from build123d import *

# Parameters (mm, degrees)
PROTO_PENTAGRAM_R   = 7.5
PROTO_PENTAGRAM_R_2 = 2.5
BOSS_EXTRUDE1_DEPTH = 15
PICK_1_R            = 1.85
CUT_EXTRUDE1_DEPTH  = 15
PICK_2_R            = 1.85
CUT_EXTRUDE2_DEPTH  = 15
PICK_3_R            = 1.85
CUT_EXTRUDE3_DEPTH  = 15
PICK_4_R            = 1.85
CUT_EXTRUDE4_DEPTH  = 15
PICK_5_R            = 1.85
CUT_EXTRUDE5_DEPTH  = 15
FILLET1_R           = 5


with BuildPart() as part:
    # proto-pentagram → Boss-Extrude1 (new body)
    # profile 1 of 2: a face of its own
    with BuildSketch(Plane(origin=(0, 0, 0), x_dir=(1, 0, 0), z_dir=(0, 1, 0))):
        Polygon((47.921856642, -22.405259561), (6.5, -8.946482483), (6.5, -52.5), (-6.5, -52.5), (-6.5, -8.946482483), (-47.921856642, -22.405259561), (-51.939077569, -10.041524849), (-10.517220927, 3.417252229), (-36.117336209, 38.652788065), (-25.600115282, 46.293996345), (0, 11.058460509), (25.600115282, 46.293996345), (36.117336209, 38.652788065), (10.517220927, 3.417252229), (51.939077569, -10.041524849), align=None)
        Circle(PROTO_PENTAGRAM_R, mode=Mode.SUBTRACT)
    # profile 2 of 2: a face of its own
    with BuildSketch(Plane(origin=(0, 0, 0), x_dir=(1, 0, 0), z_dir=(0, 1, 0))):
        Circle(PROTO_PENTAGRAM_R)
        with Locations(Location((0, 0, 0), (0, 0, 270))):
            Circle(PROTO_PENTAGRAM_R_2, mode=Mode.SUBTRACT)
    extrude(amount=BOSS_EXTRUDE1_DEPTH)

    # pick-1 → Cut-Extrude1 (cut)
    with BuildSketch(Plane(origin=(6.5, 0, 0), x_dir=(0, 0, -1), z_dir=(1, 0, 0))):
        with Locations((-46.5, 7.5)):
            Circle(PICK_1_R)
        with Locations((-32.5, 7.5)):
            Circle(PICK_1_R)
    extrude(amount=-CUT_EXTRUDE1_DEPTH, mode=Mode.SUBTRACT)

    # pick-2 → Cut-Extrude2 (cut)
    with BuildSketch(Plane(origin=(2.008610463, 0, -6.181867356), x_dir=(-0.9510565162951501, 0, -0.3090169943749584), z_dir=(0.3090169943749584, 0, -0.9510565162951501))):
        with Locations((-46.5, 7.5)):
            Circle(PICK_2_R)
        with Locations((-32.5, 7.5)):
            Circle(PICK_2_R)
    extrude(amount=-CUT_EXTRUDE2_DEPTH, mode=Mode.SUBTRACT)

    # pick-3 → Cut-Extrude3 (cut)
    with BuildSketch(Plane(origin=(-5.258610463, 0, -3.82060414), x_dir=(-0.5877852522924804, 0, 0.8090169943749422), z_dir=(-0.8090169943749423, 0, -0.5877852522924804))):
        with Locations((-46.5, 7.5)):
            Circle(PICK_3_R)
        with Locations((-32.5, 7.5)):
            Circle(PICK_3_R)
    extrude(amount=-CUT_EXTRUDE3_DEPTH, mode=Mode.SUBTRACT)

    # pick-4 → Cut-Extrude4 (cut)
    with BuildSketch(Plane(origin=(-5.258610463, 0, 3.82060414), x_dir=(0.5877852522924687, 0, 0.8090169943749507), z_dir=(-0.8090169943749508, 0, 0.5877852522924687))):
        with Locations((-46.5, 7.5)):
            Circle(PICK_4_R)
        with Locations((-32.5, 7.5)):
            Circle(PICK_4_R)
    extrude(amount=-CUT_EXTRUDE4_DEPTH, mode=Mode.SUBTRACT)

    # pick-5 → Cut-Extrude5 (cut)
    with BuildSketch(Plane(origin=(2.008610463, 0, 6.181867356), x_dir=(0.9510565162951544, 0, -0.30901699437494484), z_dir=(0.30901699437494484, 0, 0.9510565162951544))):
        with Locations((-46.5, 7.5)):
            Circle(PICK_5_R)
        with Locations((-32.5, 7.5)):
            Circle(PICK_5_R)
    extrude(amount=-CUT_EXTRUDE5_DEPTH, mode=Mode.SUBTRACT)

    # Fillet1
    fillet1_edges = [part.edges().sort_by_distance(p)[0] for p in [
        (23.317278568, 15, -21.035020147),
        (-12.800057641, 15, -28.676228427),
        (27.210928321, 15, 15.675871022),
        (-31.228149248, 15, 3.31213631),
        (-6.5, 15, 30.723241242),
    ]]
    fillet(fillet1_edges, radius=FILLET1_R)


solid = part.part
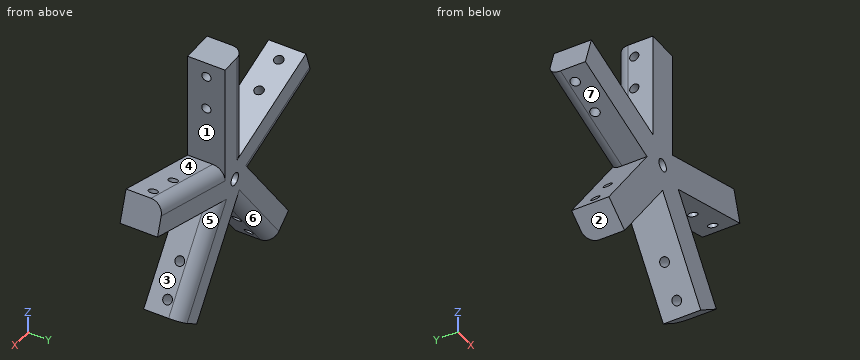
Could you check a few things on this model? Use its own coordinates, in mm. Face numbers are marked on the shaded views. A direction names the side the tool comes from. Round coordinates to 2 decimals unless told otherwise and drop trailing zeros. Order: outer loops, then holes, each group sorted by start corner. A loop starts at its lowest first (then second) coordinate and runs counter-clockwise, first axis right, second up. Notation, with made-up numbers: M -4,76 L 6,76 A28 ccw 6,107 Z; hole C 38,63.5 d11. An arc over 180 degrees is marked long. One line per item, written item: value.
(1) Which directions (+Z, -Z, +X, -X, +Y, -Y) give clear straight access to the entire face, cutting with the end or side of a thin tool? Please do the marked faces 4, 5, 6 and 7.
Ans:
face 4: +Z, +Y, -Y
face 5: +X, +Y
face 6: -Z, +Y
face 7: -X, +Y, -Y
(2) Imagine slicing it at A-A (y = 2.25). Write out the boundary of the cut face in (x, z).
Ans:
outline: M -51.94,10.04 L -10.52,-3.42 L -36.12,-38.65 L -25.6,-46.29 L 0,-11.06 L 25.6,-46.29 L 36.12,-38.65 L 10.52,-3.42 L 51.94,10.04 L 47.92,22.41 L 6.5,8.95 L 6.5,52.5 L -6.5,52.5 L -6.5,8.95 L -47.92,22.41 Z; hole C 0,0 d5
(3) I need wall thicknesses on line 1 along Y through (x, z) = (3, 46.5); line 2 along Z through (x, y) = (18.5, 8); line 3 along X through (y, z) = (1, 36). Which ranges of each line are inside material? Lowest first, please. Write a range as from..to.
Ans:
line 1: y = 0..5.65, 9.35..15
line 2: z = -36.52..-28.93, -24.53..-14.4, -0.82..12.85
line 3: x = -6.5..6.5
(4) I'm going to push flat-ended pins straight in: P1, Ø6, axis at y = 7.5, z = 32.5, coming from the -X side; P2, Ø1, axis at y = 11.5, z = -12.5, coming from the -X side; P3, Ø3, axis at x = 0, z = 0, coming from the +Y side; P4, Ø6, axis at y = 7.5, z = 46.5, coming from the +X side. Where does each tip first touch, or does it pass through?
Ans:
P1: stops at x = -6.5
P2: stops at x = -17.48
P3: passes through
P4: stops at x = 6.5
(5) If we mould it in two halves opening along Z, with no side actions, what happens to the marked faces 1, 2 and 3? For each: released by +Z, released by -Z, zero draft, split by the parting line, or undercut.
Ans:
face 1: zero draft
face 2: released by -Z
face 3: undercut
(6) Imagine slicing it at B-B (z = 32.5). Write out the boundary of the cut face in (x, y), and give its area (3 significant figures).
Ans:
outline: M -6.5,0 L 6.5,0 L 6.5,5.65 L -6.5,5.65 Z; M -6.5,9.35 L 6.5,9.35 L 6.5,15 L -1.5,15 A5 ccw -6.5,10 Z
area: 142 mm^2
(7) Imagine slicing it at C-C (y = 7.5). Count the separate pieces of the cut face and the enclosed holes in it, and give its area (3 significant figures).
Ans:
separate pieces: 11
enclosed holes: 1
area: 2,620 mm^2
